Source: CAD feature listing. Evaluate the final solid. Frame: model axes, mm. A direction names the side the tool comes from. Give positions to 0.01 mm unless a question says otherwise; leave off trailing zeros. Order: outer loops, then holes, each group sorted by start corner. A loop starts at its lowest first (then second) coordinate and runs counter-clockwise, first axis right, second up.
```python
from build123d import *

# Parameters (mm, degrees)
F2_W     = 16.304351
F2_H     = 3.93052
F3_DEPTH = 25.4
F4_R     = 1.646658
F5_DEPTH = 25.4


with BuildPart() as f1:
    # F0 (on Front) → F1 (revolve)
    with BuildSketch(Plane.XZ):
        Polygon((-52.007179, 3.804098), (-52.007179, 0), (24.581712, 0), (17.992821, 3.804098), align=None)
    revolve(axis=Axis((-13.712734, 0, 0), (1, 0, 0)))

    # F2 (on Front) → F3 (cut, symmetric)
    with BuildSketch(Plane.XZ):
        with Locations((-50.214119, 0)):
            Rectangle(F2_W, F2_H)
    extrude(amount=F3_DEPTH, both=True, mode=Mode.SUBTRACT)

    # F4 (on Top) → F5 (cut, symmetric)
    with BuildSketch(Plane.XY):
        with Locations((-46.583418, 0)):
            Circle(F4_R)
    extrude(amount=F5_DEPTH, both=True, mode=Mode.SUBTRACT)


solid = f1.part
```
1) Section query B-B, the plane y = -0.75. Count the separate pieces of the cut face and the enclosed holes in it, and give its area (3 significant figures).
Report:
separate pieces: 3
enclosed holes: 0
area: 495 mm2
2) Draft query along X for faces 1 (the flat face through (-48.2, -0.8, 1.965)), 2 (the cylindrical face through (-45.06, -0.63, 2.9)), 3 (the conical face through (21.97, 1.47, -0.33)). Return one class per face: +X half, -X half, draft (parallel to the pull), parting line (faces both ways), or undercut.
Report:
face 1: draft
face 2: undercut
face 3: +X half
3) Reachability of faces 4 (the flat face through (-52.007, 0, 3)), 5 (the flat face through (-48.2, -0.8, -1.965)) from +Z, -Z, +X, -X, +Y, -Y: full face, straight path, thin tool, end or side. Return the list, or none.
Report:
face 4: +Z, -Z, -X, +Y, -Y
face 5: -X, +Y, -Y
4) Material intervals for L1, parallel to Y at x = -4.5, z = -3.25; L2, parallel to X at y = -0.75, z = -3; L3, parallel to X at y = 0, z = 3.45, sorted ascending.
Report:
L1: y = -1.98 to 1.98
L2: x = -52.01 to -48.05, -45.12 to 19.23
L3: x = -52.01 to -48.23, -44.94 to 18.61
5) Pin query (flat end, axial travel): pin 1 (4 mm diameter, centred on x = -23, y = -3, fed in from +Z); pin 2 (1.2 mm diameter, centred on y = -1.5, z = -0.5, fed in from -X); pin 3 (1 mm diameter, centred on x = -37, y = -3, fed in from +Z). Return the tip coordinate at first contact, or that it passes through.
Report:
pin 1: stops at z = 3.67
pin 2: stops at x = -42.06
pin 3: stops at z = 2.87
6) Section query A-A, the plane x = 2. Return the cut outline in (y, z), and give its area (3 significant figures).
Report:
outline: circle Ø7.61 at (0, 0)
area: 45.5 mm2
